Could you check a few things on this model? Use its own coordinates, in mm. A direction names the side the tool comes from. Round coordinates to 2 decimals unless told otherwise and drop trailing zeros. Loops run counter-clockwise (first coordinate to the right, second up) from the corner with the lowest first, then second, coordinate; pieces in that order, holes last. Notation, with made-up numbers: M 48,58 L 77,58 A20 cw 77,63 Z; hole C -32,37.25 d9. An arc over 180 degrees is marked long. Answer in a Markdown table with one row per item.
```python
from build123d import *

# Parameters (mm, degrees)
F1_DEPTH  = 5.715
F2_R      = 10.8839
F3_DEPTH  = 25.4
F4_W      = 5.715
F4_H      = 21.9964
F5_DEPTH  = 10.16
F6_R      = 5.07999
F7_R      = 5.08
F8_W      = 5.715
F8_H      = 21.9964
F9_DEPTH  = 10.16
F10_R     = 5.07999
F11_W     = 21.9964
F11_H     = 5.715
F12_DEPTH = 10.16
F13_R     = 5.07999
F14_R     = 10.9982
F15_DEPTH = 25.4


# Not quite as in the source:
# - a fillet or chamfer is up to 0.001 mm smaller than in the source, because OpenCascade refuses the exact size


with BuildPart() as f1:
    # F0 (on Front) → F1 (new body)
    with BuildSketch(Plane.XZ):
        Polygon((-50.8, -29.3293936748), (50.8, -29.3293936748), (0, 58.6587873497), align=None)
    extrude(amount=F1_DEPTH)

    # F2 (on face) → F3 (cut)
    with BuildSketch(Plane.XZ.offset(5.715)):
        Circle(F2_R)
    extrude(amount=-F3_DEPTH, mode=Mode.SUBTRACT)

    # F4 (on face) → F5 (cut)
    with BuildSketch(Plane(origin=(25.4, 0, 14.6646968374), x_dir=(0, 1, 0), z_dir=(0.8660254038, 0, 0.5))):
        with Locations((-2.8575, 0.9615815512)):
            Rectangle(F4_W, F4_H)
    extrude(amount=-F5_DEPTH, mode=Mode.SUBTRACT)

    # F6 (radius 5.08 in the source; OpenCascade refuses exactly that, so slightly less here)
    f6_edges = [f1.edges().sort_by_distance(p)[0] for p in [
        (21.619491, -2.8575, 0.89273),
        (10.621291, -2.8575, 19.942171),
        (30.418309, -2.8575, 5.97273),
        (19.420109, -2.8575, 25.022171),
    ]]
    fillet(f6_edges, radius=F6_R)

    # F7
    f7_edges = [f1.edges().sort_by_distance(p)[0] for p in [
        (50.8, -2.8575, -29.329394),
        (-50.8, -2.8575, -29.329394),
        (0, -2.8575, 58.658787),
    ]]
    fillet(f7_edges, radius=F7_R)

    # F8 (on face) → F9 (cut)
    with BuildSketch(Plane(origin=(-25.4, 0, 14.6646968374), x_dir=(0, -1, 0), z_dir=(-0.8660254038, 0, 0.5))):
        with Locations((2.8575, -2.5338024565)):
            Rectangle(F8_W, F8_H)
    extrude(amount=-F9_DEPTH, mode=Mode.SUBTRACT)

    # F10 (radius 5.08 in the source; OpenCascade refuses exactly that, so slightly less here)
    f10_edges = [f1.edges().sort_by_distance(p)[0] for p in [
        (-21.167801, -2.8575, 21.99508),
        (-12.368983, -2.8575, 16.91508),
        (-32.166001, -2.8575, 2.945639),
        (-23.367183, -2.8575, -2.134361),
    ]]
    fillet(f10_edges, radius=F10_R)

    # F11 (on face) → F12 (cut)
    with BuildSketch(Plane(origin=(0, 0, -29.3293936748), x_dir=(1, 0, 0), z_dir=(0, 0, -1))):
        with Locations((0.2968947671, 2.8575)):
            Rectangle(F11_W, F11_H)
    extrude(amount=-F12_DEPTH, mode=Mode.SUBTRACT)

    # F13 (radius 5.08 in the source; OpenCascade refuses exactly that, so slightly less here)
    f13_edges = [f1.edges().sort_by_distance(p)[0] for p in [
        (11.295095, -2.8575, -29.329394),
        (11.295095, -2.8575, -19.169394),
        (-10.701305, -2.8575, -29.329394),
        (-10.701305, -2.8575, -19.169394),
    ]]
    fillet(f13_edges, radius=F13_R)

    # F14 (on face) → F15 (cut)
    with BuildSketch(Plane(origin=(0, 0, 0), x_dir=(-1, 0, 0), z_dir=(0, 1, 0))):
        with Locations((0, 28.7260549402)):
            Circle(F14_R)
        with Locations((25.8424041398, -15.1333886554)):
            Circle(F14_R)
        with Locations((-24.7085423876, -14.9420522576)):
            Circle(F14_R)
    extrude(amount=-F15_DEPTH, mode=Mode.SUBTRACT)


solid = f1.part
```
1) If we mould it in two halves opening along Z, with no side actions, what happens to faces 4 (the face through (-36.333, -2.817, -11.83)), 5 (the face through (-29, -3, -29.329)), 6 (the face through (-11, 0, -3)), 7 (the face through (-31.675, -2.898, 0.898))? For each: released by +Z, released by -Z, zero draft, split by the parting line, or undercut.
Computed:
| item | result |
|---|---|
| face 4 | undercut |
| face 5 | released by -Z |
| face 6 | zero draft |
| face 7 | released by +Z |
2) I want a section at D-D, the plane z = -23. Please give me the cut outline in (x, y) (3 decimals), plus the area to 3 significant figures.
Computed:
| item | result |
|---|---|
| outline | M -46.925,-5.715 L -33.529,-5.715 L -33.529,0 L -46.925,0 Z; M -18.156,-5.715 L -10.545,-5.715 L -10.545,0 L -18.156,0 Z; M 11.139,-5.715 L 17.223,-5.715 L 17.223,0 L 11.139,0 Z; M 32.194,-5.715 L 46.925,-5.715 L 46.925,0 L 32.194,0 Z |
| area | 239 mm² |
3) I want a section at B-B, the plane z = 30.5. Please give me the cut outline in (x, y) (3 decimals).
Computed:
| item | result |
|---|---|
| outline | M -16.257,-5.715 L -10.854,-5.715 L -10.854,0 L -16.257,0 Z; M 10.854,-5.715 L 16.257,-5.715 L 16.257,0 L 10.854,0 Z |
4) I want a section at A-A, the plane x = 0. Please give me the cut outline in (y, z) (3 decimals), plus the area to 3 significant figures.
Computed:
| item | result |
|---|---|
| outline | M -5.715,-19.169 L 0,-19.169 L 0,-10.884 L -5.715,-10.884 Z; M -5.715,10.884 L 0,10.884 L 0,17.728 L -5.715,17.728 Z; M -5.715,39.724 L 0,39.724 L 0,53.579 L -5.715,53.579 Z |
| area | 166 mm² |
5) I need wall thicknesses on line 1 (Z direction, x = 0, y = -4.4); line 2 (X direction, y = -2.1, z = -5); line 3 (X direction, y = -4.7, z = -17). Which ranges of each line are inside material? Lowest first, please.
Computed:
| item | result |
|---|---|
| line 1 | z = -19.17 to -10.88, 10.88 to 17.73, 39.72 to 53.58 |
| line 2 | x = -36.75 to -30.12, -21.57 to -9.67, 9.67 to 20.01, 29.41 to 36.75 |
| line 3 | x = -43.68 to -36.68, -15 to 13.9, 35.51 to 43.68 |
6) Will these pins go through, and if not, where does the flat tip stop? P1, Ø3, axis at x = 37, y = -3.5, coming from the +Z side; P2, Ø12, axis at x = -32, z = -10.5, coming from the -Y side (3 decimals); P3, Ø1.5, axis at y = -1.5, z = 36, coming from the +X side; P4, Ø3, axis at x = 1.5, y = -4, coming from the -Z side.
Computed:
| item | result |
|---|---|
| P1 | stops at z = -2.83 |
| P2 | stops at y = -5.715 |
| P3 | stops at x = 13.52 |
| P4 | stops at z = -19.17 |
7) I want a section at C-C, the plane y = -1.6. State how many separate pieces and enclosed holes the cut face has, plus the area to 3 significant figures.
Computed:
| item | result |
|---|---|
| separate pieces | 1 |
| enclosed holes | 4 |
| area | 2,230 mm² |
8) Which directions (+Z, -Z, +X, -X, +Y, -Y) give clear straight access to the entire face, cutting with the end or side of a thin tool? Please do faces 1 (the face through (-17.83, -2.82, 7.46)), 2 (the face through (12.82, -2.9, -27.88)), 3 (the face through (-11.414, -2.817, 38.889)).
Computed:
| item | result |
|---|---|
| face 1 | -X, +Y, -Y |
| face 2 | -Z, +Y, -Y |
| face 3 | +Z, -X, +Y, -Y |
